Answer from the drawing. Dimensions are ordinates in mm from the lowest x, y and z of the part. A direction names the side the tool comes from. Coordinates: 2 decimals unless noted, no trailing zeros. Write each loop counter-clockwise with the first axis right and the second up, starting at its lowest first coordinate (ties: lowest second). Pieces come first, ordered by that corner, then holes.
(1) Section C-C on y = 142 is taken. Write down the section's boundary in (x, z) (1 decimal).
(2) Given pin 1 (3 mm diameter, centred on x = 12, z = 28.5, fed in from +Y); pin 2 (5 mm diameter, centred on x = 28.5, y = 130, fed in from -Z) (1 decimal); pin 3 (6 mm diameter, centred on y = 132.5, z = 18, fed in from -X), each flat-ended and moving along its own axis, determine where each tip first touches the part or whether it passes through.
(3) Section B-B on x = 17 is taken. Write down the section's boundary in (y, z), then the cut area to 3 significant figures.
(4) Find the intervals of material crossed by probe 1 along Y at (x, z) = (5, 17); probe 2 along X at (y, z) = (132, 26); probe 3 along Z at (x, y) = (3.5, 142), in increasing order.
(5) Section D-D on x = 4.5 is taken. Write down the section's boundary in (y, z) (1 decimal), then the cut area to 3 significant figures.
(6) The mould has two halves that part along X. Classify the marked faces 3, 4 and 5: +X half, -X half, draft (parallel to the pull), parting line (faces both ways), or undercut.
(7) Section A-A on z = 17 is taken. Write down the section's boundary in (x, y), then the cut area to 3 significant figures.
(8) Which of the six approach directions +Z, -Z, +X, -X, +Y, -Y give full straight-line access (tool end or side, diameter ignored) to the marked faces 1 and 2?
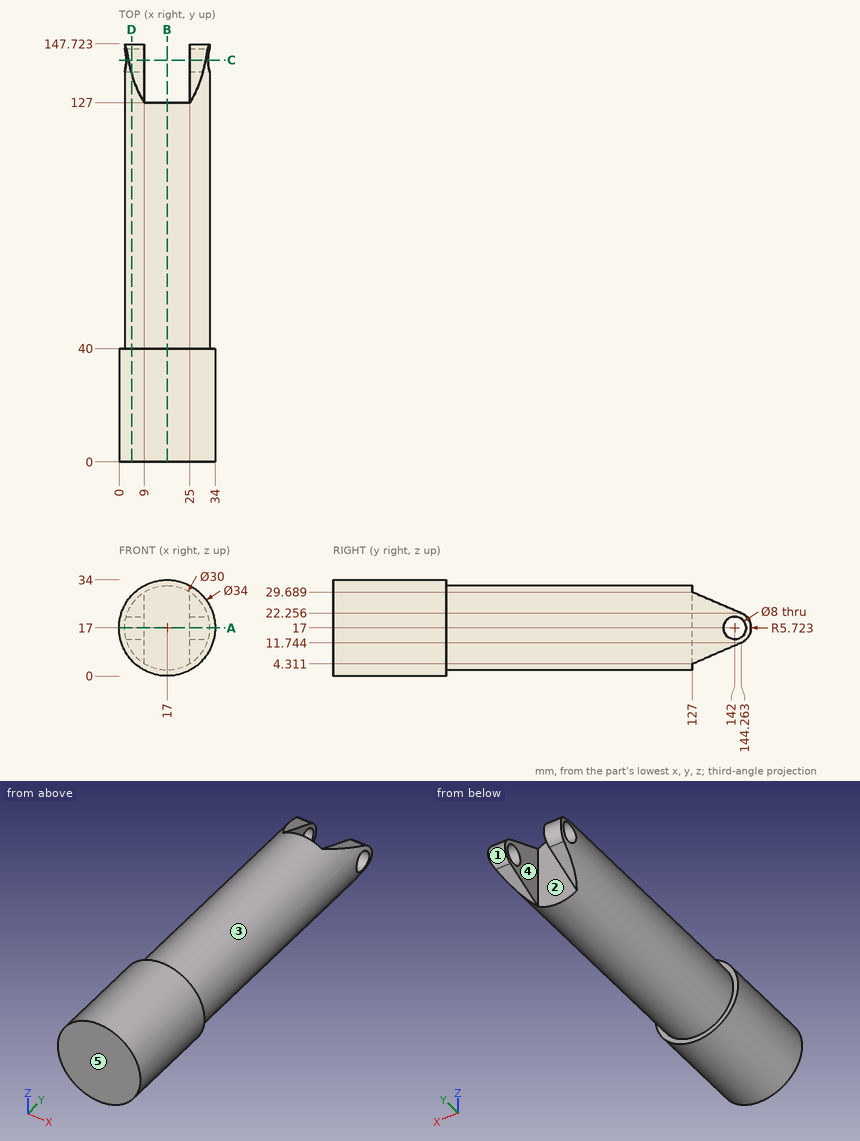
Response:
1. outline: (2.5, 13) arc R15 ccw to (3.4, 10.8) - (9, 10.8) - (9, 13) - close; (2.5, 21) - (9, 21) - (9, 23.2) - (3.4, 23.2) arc R15 ccw to start; (25, 10.8) - (30.6, 10.8) arc R15 ccw to (31.5, 13) - (25, 13) - close; (25, 21) - (31.5, 21) arc R15 ccw to (30.6, 23.2) - (25, 23.2) - close
2. pin 1: stops at y = 127
2. pin 2: stops at z = 5.2
2. pin 3: stops at x = 2
3. outline: (0, 0) - (40, 0) - (40, 2) - (127, 2) - (127, 32) - (40, 32) - (40, 34) - (0, 34) - close
3. area: 3,970 mm2
4. probe 1: y = 0 to 138, 146 to 147.72
4. probe 2: x = 5 to 9, 25 to 29
4. probe 3: z = 10.77 to 13, 21 to 23.23
5. outline: (0, 5.5) - (40, 5.5) - (40, 8.7) - (137.2, 8.7) - (144.3, 11.7) arc R5.7 ccw to (144.3, 22.3) - (137.2, 25.3) - (40, 25.3) - (40, 28.5) - (0, 28.5) - close; hole circle Ø8 at (142, 17)
5. area: 2,610 mm2
6. face 3: parting line
6. face 4: undercut
6. face 5: draft
7. outline: (0, 0) - (34, 0) - (34, 40) - (32, 40) - (32, 138) - (25, 138) - (25, 127) - (9, 127) - (9, 138) - (2, 138) - (2, 40) - (0, 40) - close; (2, 146) - (9, 146) - (9, 147.72) - (2, 147.72) - close; (25, 146) - (32, 146) - (32, 147.72) - (25, 147.72) - close
7. area: 4,150 mm2
8. face 1: +X, -X, +Y
8. face 2: +Z, -Z, +Y
